from build123d import *

# Parameters (mm, degrees)
F0_R     = 15.6
F0_R_2   = 5.6
F0_R_3   = 3.9
F1_DEPTH = 3
F2_DEPTH = 4
F3_DEPTH = 8
F4_R     = 2


# Not quite as in the source:
# - a fillet or chamfer that OpenCascade refuses, or shapes differently, is made with other operations: its cross-section is extruded or revolved along the edge and cut away or added


with BuildPart() as f1:
    # F0 (on Top) → F1 (new body)
    with BuildSketch(Plane.XY):
        Circle(F0_R)
        Circle(F0_R_2, mode=Mode.SUBTRACT)
        Circle(F0_R_2)
        Circle(F0_R_3, mode=Mode.SUBTRACT)
        Circle(F0_R_3)
    extrude(amount=-F1_DEPTH)

    # F0 (on Top) → F2 (join)
    with BuildSketch(Plane.XY):
        Circle(F0_R_2)
        Circle(F0_R_3, mode=Mode.SUBTRACT)
        Circle(F0_R_3)
    extrude(amount=-F2_DEPTH)

    # F0 (on Top) → F3 (join)
    with BuildSketch(Plane.XY):
        Circle(F0_R_3)
    extrude(amount=-F3_DEPTH)

    # F4
    f4_edges = [f1.edges().sort_by_distance(p)[0] for p in [
        (-15.6, 0, -3),
    ]]
    fillet(f4_edges, radius=F4_R)

    # F5: fillet of radius 2 on 1 edges, made by hand

    # F5_s1 → F5_t2 (revolve, cut)
    with BuildSketch(Plane.XZ):
        with BuildLine():
            ThreePointArc((15.6, -1), (14.8679491924, -0.2679491924), (13.8679491924, 0))
            Line((13.8679491924, 0), (15.6, 0))
            Line((15.6, 0), (15.6, -1))
        make_face()
    revolve(axis=Axis((0, 0, 0), (0, 0, 1)), mode=Mode.SUBTRACT)


solid = f1.part
The listing builds one solid part. Answer for the finished solid, in the listing's coordinates (mm). A direction names the side the tool comes from. Coordinates: 2 decimals unless noted, no trailing zeros. Order: outer loops, then holes, each group sorted by start corner. A loop starts at its lowest first (then second) coordinate and runs counter-clockwise, first axis right, second up. Notation, with made-up numbers: (-13.5, -37) -> (3.5, -37) arc R25 cw to (3.5, -25) -> close; hole circle Ø7 at (-23, -37.75). An arc over 180 degrees is marked (long way). Answer in a Markdown table with one row per item. Add a question column.
Item 1: Each of these flat-tipped pins is pushed along its axis until it touches: P1, Ø4, axis at x = 9, z = -2.5, coming from the +Y side; P2, Ø1.5, axis at y = 1, z = -5.5, coming from the +X side; P3, Ø1.5, axis at x = -6.5, z = -2.5, coming from the +Y side. Where does it stop, or does it pass through?
Item 2: Find section D-D (z = -2.5). Write down the section's boundary in (x, y), then the cut area to 3 significant figures.
Item 3: Find section A-A (x = 0). Write down the section's boundary in (y, z).
Item 4: Find section C-C (z = -6.25). Write down the section's boundary in (x, y), then the cut area to 3 significant figures.
Item 5: Find the intervals of material crossed by L1, parallel to Z at x = -11.5, y = -1.5; L2, parallel to Y at x = -1.5, z = -5, in increasing order. Write a range as from..to.
Item 6: Which of the six approach directions +Z, -Z, +X, -X, +Y, -Y give full straight-line access (tool end or side, diameter ignored) to faces 1 (the face through (0, 0, -8)), 2 (the face through (-4, -1, -4))?
Result set:
| question | item | result |
|---|---|---|
| 1 | P1 | stops at y = 13.73 |
| 1 | P2 | stops at x = 3.89 |
| 1 | P3 | stops at y = 14.15 |
| 2 | outline | circle Ø29.85 at (0, 0) |
| 2 | area | 700 mm² |
| 3 | outline | (-15.6, -1) arc R2 ccw to (-13.6, -3) -> (-5.6, -3) -> (-5.6, -4) -> (-3.9, -4) -> (-3.9, -8) -> (3.9, -8) -> (3.9, -4) -> (5.6, -4) -> (5.6, -3) -> (13.6, -3) arc R2 ccw to (15.6, -1) arc R2 ccw to (13.87, 0) -> (-13.87, 0) arc R2 ccw to start |
| 4 | outline | circle Ø7.8 at (0, 0) |
| 4 | area | 47.8 mm² |
| 5 | L1 | z = -3..0 |
| 5 | L2 | y = -3.6..3.6 |
| 6 | face 1 | -Z, +X, -X, +Y, -Y |
| 6 | face 2 | -Z |
